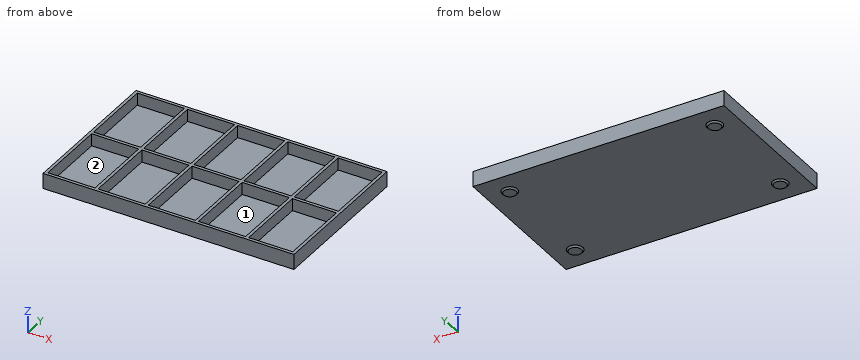
```python
from build123d import *

# Parameters (mm, degrees)
F0_W     = 164
F0_H     = 101
F1_DEPTH = 10
F2_W     = 160
F2_H     = 97
F3_DEPTH = 8
F4_W     = 160
F4_H     = 2
F5_DEPTH = 8
F6_W     = 2
F6_H     = 97
F7_DEPTH = 8
F8_R     = 5
F9_DEPTH = 1
F10_SIZE = 0.99999


# Not quite as in the source:
# - a fillet or chamfer is up to 0.001 mm smaller than in the source, because OpenCascade refuses the exact size


with BuildPart() as f1:
    # F0 (on Top) → F1 (new body)
    with BuildSketch(Plane.XY):
        Rectangle(F0_W, F0_H)
    extrude(amount=F1_DEPTH)

    # F2 (on face) → F3 (cut)
    with BuildSketch(Plane.XY.offset(10)):
        Rectangle(F2_W, F2_H)
    extrude(amount=-F3_DEPTH, mode=Mode.SUBTRACT)

    # F4 (on face) → F5 (join)
    with BuildSketch(Plane.XY.offset(2)):
        Rectangle(F4_W, F4_H)
    extrude(amount=F5_DEPTH)

    # F6 (on face) → F7 (join)
    with BuildSketch(Plane.XY.offset(2)):
        with Locations((-48.2, 0)):
            Rectangle(F6_W, F6_H)
        with Locations((-15.4, 0)):
            Rectangle(F6_W, F6_H)
        with Locations((17.4, 0)):
            Rectangle(F6_W, F6_H)
        with Locations((50.2, 0)):
            Rectangle(F6_W, F6_H)
    extrude(amount=F7_DEPTH)

    # F8 (on face) → F9 (join)
    with BuildSketch(Plane(origin=(0, 0, 0), x_dir=(1, 0, 0), z_dir=(0, 0, -1))):
        with Locations((-67, 35.5)):
            Circle(F8_R)
        with Locations((67, 35.5)):
            Circle(F8_R)
        with Locations((67, -35.5)):
            Circle(F8_R)
        with Locations((-67, -35.5)):
            Circle(F8_R)
    extrude(amount=F9_DEPTH)

    # F10 (size 1 in the source; OpenCascade refuses exactly that, so slightly less here)
    f10_edges = [f1.edges().sort_by_distance(p)[0] for p in [
        (-72, -35.5, -1),
        (-72, 35.5, -1),
        (62, -35.5, -1),
        (62, 35.5, -1),
    ]]
    chamfer(f10_edges, length=F10_SIZE)


solid = f1.part
```
CAD build for the part. Positions are in the model's coordinates, mm. Face numbers are marked on the shaded views. Coordinates: 2 decimals unless noted, no trailing zeros. Write each loop counter-clockwise with the first axis right and the second up, starting at its lowest first coordinate (ties: lowest second). Pieces come first, ordered by that corner, then holes.
(1) Cut at C-C, the plane z = 3.75. Count the separate pieces of the cut face and the enclosed holes in it, and give its area (3 significant figures).
(2) Cut at B-B, the plane y = -9. List the corners of the cut face in (x, z).
(3) Cut at A-A, the plane x = -24. List the corners of the cut face in (y, z), and give its area (3 significant figures).
(4) Flat gauge pin, fed straight in: pin 1 (1 mm diameter, centred on x = -8.5, y = 4.5, fed in from +Z). Where does the tip first touch, or does it go through?
(5) Two-plate mould, pull along X, no slides. Class the marked faces 1 and 2: +X half, -X half, draft (parallel to the pull), parting line (faces both ways), or undercut.
(6) Drill centre lines: probe 1 along Y at (x, z) = (-46.5, 9); probe 2 along X at (y, z) = (21.5, 3.25); probe 3 along Z at (x, y) = (10.5, 34.5). Where is each one in solid material? Low to high.
Geometry says:
1. separate pieces: 1
1. enclosed holes: 10
1. area: 2,120 mm2
2. outline: (-82, 0) - (82, 0) - (82, 10) - (80, 10) - (80, 2) - (51.2, 2) - (51.2, 10) - (49.2, 10) - (49.2, 2) - (18.4, 2) - (18.4, 10) - (16.4, 10) - (16.4, 2) - (-14.4, 2) - (-14.4, 10) - (-16.4, 10) - (-16.4, 2) - (-47.2, 2) - (-47.2, 10) - (-49.2, 10) - (-49.2, 2) - (-80, 2) - (-80, 10) - (-82, 10) - close
3. outline: (-50.5, 0) - (50.5, 0) - (50.5, 10) - (48.5, 10) - (48.5, 2) - (1, 2) - (1, 10) - (-1, 10) - (-1, 2) - (-48.5, 2) - (-48.5, 10) - (-50.5, 10) - close
3. area: 250 mm2
4. pin 1: stops at z = 2
5. face 1: undercut
5. face 2: undercut
6. probe 1: y = -50.5 to -48.5, -1 to 1, 48.5 to 50.5
6. probe 2: x = -82 to -80, -49.2 to -47.2, -16.4 to -14.4, 16.4 to 18.4, 49.2 to 51.2, 80 to 82
6. probe 3: z = 0 to 2
